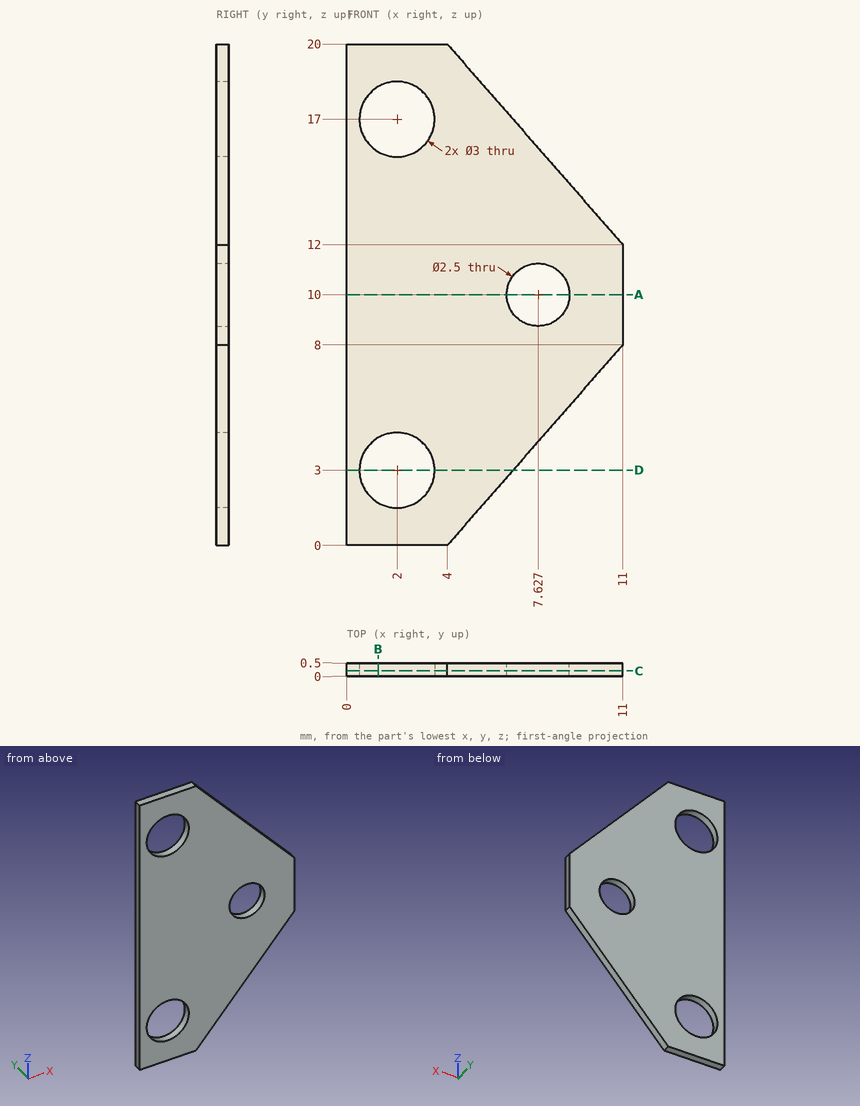
Check sheet for the drawn part. Datum: minimum x, y, z corner. Units: mm. Give positions to 0.01 mm unless a question says otherwise; leave off trailing zeros. Order: outer loops, then holes, each group sorted by start corner. A loop starts at its lowest first (then second) coordinate and runs counter-clockwise, first axis right, second up. Notation, with made-up numbers: (20.25, 74) - (76.25, 74) arc R16 cw to (76.25, 96) - close; hole circle Ø6 at (54, 28). An arc over 180 degrees is marked (long way). Answer in a Markdown table with one row per item. Add a question column.
Q1. Cross-section at D-D, the plane z = 3. Enter the section's corners in (x, y) (1 decimal).
Q2. Cross-section at C-C, the plane y = 0.2. Enter the section's corners in (x, z), then the cut area to 3 significant figures.
Q3. Material ranges on probe 1 along Z at (x, y) = (1.25, 0.2); probe 2 along Z at (x, y) = (8.5, 0.15) (1 decimal); probe 3 along Z at (x, y) = (8, 0.2) (1 decimal), recorded low to high. Write a range as from..to.
Q4. Cross-section at A-A, the plane z = 10. Enter the section's corners in (x, y).
Q5. Cross-section at B-B, the plane x = 1.25. Enter the section's corners in (y, z).
Check values:
| question | item | result |
|---|---|---|
| 1 | outline | (0, 0) - (0.5, 0) - (0.5, 0.5) - (0, 0.5) - close; (3.5, 0) - (6.6, 0) - (6.6, 0.5) - (3.5, 0.5) - close |
| 2 | outline | (0, 0) - (4, 0) - (11, 8) - (11, 12) - (4, 20) - (0, 20) - close; hole circle Ø3 at (2, 3); hole circle Ø3 at (2, 17); hole circle Ø2.5 at (7.63, 10) |
| 2 | area | 145 mm^2 |
| 3 | probe 1 | z = 0..1.7, 4.3..15.7, 18.3..20 |
| 3 | probe 2 | z = 5.1..9.1, 10.9..14.9 |
| 3 | probe 3 | z = 4.6..8.8, 11.2..15.4 |
| 4 | outline | (0, 0) - (6.38, 0) - (6.38, 0.5) - (0, 0.5) - close; (8.88, 0) - (11, 0) - (11, 0.5) - (8.88, 0.5) - close |
| 5 | outline | (0, 0) - (0.5, 0) - (0.5, 1.7) - (0, 1.7) - close; (0, 4.3) - (0.5, 4.3) - (0.5, 15.7) - (0, 15.7) - close; (0, 18.3) - (0.5, 18.3) - (0.5, 20) - (0, 20) - close |
